The listing builds one solid part. Answer for the finished solid, in the listing's coordinates (mm). Give positions to 0.01 mm unless a question says otherwise; leave off trailing zeros. Write each loop counter-clockwise with the first axis right and the second up, starting at its lowest first coordinate (ties: lowest second). Pieces come first, ordered by that corner, then holes. Notation, with made-up numbers: (-21.5, -14.75) - (-0.5, -14.75) arc R14 cw to (-0.5, -10.75) - close; hole circle Ø4 at (11, -39). An arc over 180 degrees is marked (long way). One line per item, written item: value. Start each with the question number.
from build123d import *

# Parameters (mm, degrees)
SKETCH_1_R      = 3
SKETCH_1_R_2    = 1.5
EXTRUDE_1_DEPTH = 1.5


with BuildPart() as part:
    # 草图1 → 凸台-拉伸1 (new body)
    with BuildSketch(Plane.XY):
        with BuildLine():
            Line((-25.801260856, 11.030846734), (34.198739144, 11.030846734))
            Line((34.198739144, 11.030846734), (44.198739144, 11.030846734))
            ThreePointArc((44.198739144, 11.030846734), (47.027166269, 9.859273858), (48.198739144, 7.030846734))
            Line((48.198739144, 7.030846734), (48.198739144, -14.969153266))
            ThreePointArc((48.198739144, -14.969153266), (47.027166269, -17.797580391), (44.198739144, -18.969153266))
            Line((44.198739144, -18.969153266), (34.198739144, -18.969153266))
            Line((34.198739144, -18.969153266), (-25.801260856, -18.969153266))
            Line((-25.801260856, -18.969153266), (-35.801260856, -18.969153266))
            ThreePointArc((-35.801260856, -18.969153266), (-38.62968798, -17.797580391), (-39.801260856, -14.969153266))
            Line((-39.801260856, -14.969153266), (-39.801260856, 7.030846734))
            ThreePointArc((-39.801260856, 7.030846734), (-38.62968798, 9.859273858), (-35.801260856, 11.030846734))
            Line((-35.801260856, 11.030846734), (-25.801260856, 11.030846734))
        make_face()
        with Locations((4.198739144, -9.469153266)):
            Circle(SKETCH_1_R, mode=Mode.SUBTRACT)
        with Locations((-17.801260856, 6.030846734)):
            Circle(SKETCH_1_R_2, mode=Mode.SUBTRACT)
        with Locations((-33.801260856, 6.030846734)):
            Circle(SKETCH_1_R_2, mode=Mode.SUBTRACT)
        with Locations((26.198739144, 6.030846734)):
            Circle(SKETCH_1_R_2, mode=Mode.SUBTRACT)
        with Locations((42.198739144, 6.030846734)):
            Circle(SKETCH_1_R_2, mode=Mode.SUBTRACT)
    extrude(amount=EXTRUDE_1_DEPTH)


solid = part.part
Item 1: The mould has two halves that part along Y. Classify faces 1 (the cylindrical face through (46.996, 9.89, 0.74)), 2 (the flat face through (5, -4, 0)), 3 (the cylindrical face through (3.55, -12.4, 0.74)), 4 (the cylindrical face through (-38.598, -17.829, 0.74)): +Y half, -Y half, draft (parallel to the pull), parting line (faces both ways), or undercut.
Item 2: Find section A-A on z = 0.5. Determine the outline of the cut face in (x, y).
Item 3: Straight lines are drawn through the part: line 1 along X through (y, z) = (7, 0.4); line 2 along X through (y, z) = (-9.5, 1.4); line 3 along Y through (x, z) = (-34, 1). For each, find the intervals that lie inside material, in ascending order.
Item 4: Find section B-B on y = -8.5. Determine the outline of the cut face in (x, z), plus the area to 3 significant figures.
Values:
1. face 1: +Y half
1. face 2: draft
1. face 3: undercut
1. face 4: -Y half
2. outline: (-39.8, -14.97) arc R4 ccw to (-35.8, -18.97) - (44.2, -18.97) arc R4 ccw to (48.2, -14.97) - (48.2, 7.03) arc R4 ccw to (44.2, 11.03) - (-35.8, 11.03) arc R4 ccw to (-39.8, 7.03) - close; hole circle Ø3 at (-33.8, 6.03); hole circle Ø3 at (-17.8, 6.03); hole circle Ø6 at (4.2, -9.47); hole circle Ø3 at (26.2, 6.03); hole circle Ø3 at (42.2, 6.03)
3. line 1: -39.8 to -34.95, -32.66 to -18.95, -16.66 to 25.05, 27.34 to 41.05, 43.34 to 48.2
3. line 2: -39.8 to 1.2, 7.2 to 48.2
3. line 3: -18.97 to 4.54, 7.52 to 11.03
4. outline: (-39.8, 0) - (1.36, 0) - (1.36, 1.5) - (-39.8, 1.5) - close; (7.04, 0) - (48.2, 0) - (48.2, 1.5) - (7.04, 1.5) - close
4. area: 123 mm^2
